Model file for the job. Use its own axes, mm. Face numbers are marked on the shaded views. A direction names the side the tool comes from. Coordinates: 2 decimals unless noted, no trailing zeros. Write each loop counter-clockwise with the first axis right and the second up, starting at its lowest first coordinate (ties: lowest second). Pieces come first, ordered by that corner, then holes. Notation, with made-up numbers: M 69.25,85 L 116.25,85 A25 ccw 116.25,100 Z; hole C -37.5,-13 d9. An arc over 180 degrees is marked long. Answer in a Markdown table with one row per item. Add a question column.
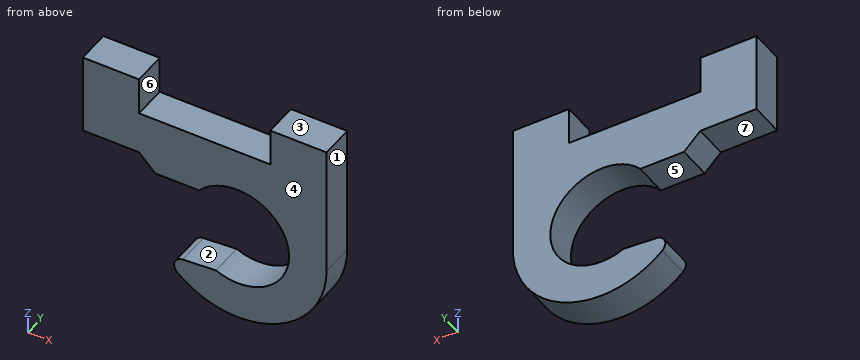
```python
from build123d import *

# Parameters (mm, degrees)
SKETCH1_R           = 2.75
BOSS_EXTRUDE1_DEPTH = 1.8
CUT_EXTRUDE1_DEPTH  = 1.8
FILLET1_R           = 0.5


with BuildPart() as part:
    # Sketch1 → Boss-Extrude1 (new body)
    with BuildSketch(Plane(origin=(0, 0, 0), x_dir=(1, 0, 0), z_dir=(0, 1, 0))):
        with BuildLine():
            Line((4.75, 0), (4.75, -5))
            Line((4.75, -5), (4.75, -7))
            Line((4.75, -7), (1.75, -7))
            Line((1.75, -7), (1.75, -5))
            Line((1.75, -5), (-5.25, -5))
            Line((-5.25, -5), (-5.25, -7))
            Line((-5.25, -7), (-8.25, -7))
            Line((-8.25, -7), (-8.25, -5))
            Line((-8.25, -5), (-8.25, -2.7))
            Line((-8.25, -2.7), (-5.25, -2.7))
            Line((-5.25, -2.7), (-4.382350157, -1.832350157))
            ThreePointArc((-4.382350157, -1.832350157), (-0.93443479, 4.657180652), (4.75, 0))
        make_face()
        Circle(SKETCH1_R, mode=Mode.SUBTRACT)
    extrude(amount=BOSS_EXTRUDE1_DEPTH)

    # Sketch2 → Cut-Extrude1 (cut)
    with BuildSketch(Plane(origin=(0, 1.8, 0), x_dir=(1, 0, 0), z_dir=(0, 1, 0))):
        Polygon((-5, 2.767649843), (0, 2.418015783), (0, -1.832350157), (-5, -1.832350157), align=None)
    extrude(amount=-CUT_EXTRUDE1_DEPTH, mode=Mode.SUBTRACT)

    # Fillet1
    fillet1_edges = [part.edges().sort_by_distance(p)[0] for p in [
        (-3.913732442, 0.9, -2.691690615),
    ]]
    fillet(fillet1_edges, radius=FILLET1_R)


solid = part.part
```
1) Drill centre lines: probe 1 along Z at (x, y) = (0, 1.2); probe 2 along X at (y, z) = (1.05, 0); probe 3 along Z at (x, y) = (-4, 0.25). Where is each one in solid material? Low to high.
2) Two-plate mould, pull along Z, no slides. Class the marked faces 1, 2 and 3: released by +Z, released by -Z, zero draft, split by the parting line, or undercut.
3) Slice it at C-C (y = 0.85). Give the cut face in (x, z), then the cut area to 3 significant figures.
4) Which spindle directions (+Z, -Z, +X, -X, +Y, -Y) get a long thin tool onto all of the face, cutting with end or side? Do the marked faces 4, 5, 6 and 7. Say none if no direction does.
5) Flat gauge pins, fed straight in: pin 1 Ø0.5 at (x, y) = (-3, 1) entering from -Z; pin 2 Ø3.5 at (x, z) = (0, 0) entering from +Y; pin 3 Ø0.5 at (x, y) = (-1.5, 1) entering from +Z; pin 4 Ø0.9 at (x, y) = (-7, 1) entering from -Z. Where does each tip first touch, or does it go through?
6) Slice it at A-A (z = 6). Give the cut face in (x, y).
7) Slice it at D-D (x = 3.25). Give the cut face in (y, z).
8) Slice it at B-B (x = 0). Give the cut face in (y, z), then the cut area to 3 significant figures.
Ans:
| question | item | result |
|---|---|---|
| 1 | probe 1 | z = -4.75 to -2.75, 2.75 to 5 |
| 1 | probe 2 | x = 2.75 to 4.75 |
| 1 | probe 3 | z = 1.83 to 5 |
| 2 | face 1 | zero draft |
| 2 | face 2 | undercut |
| 2 | face 3 | released by +Z |
| 3 | outline | M -8.25,2.7 L -5.25,2.7 L -4.38,1.83 L -2.05,1.83 A2.75 cw long -1.15,-2.5 L -2.92,-2.62 A0.5 ccw -3.22,-3.49 A4.75 ccw 4.75,0 L 4.75,7 L 1.75,7 L 1.75,5 L -5.25,5 L -5.25,7 L -8.25,7 Z |
| 3 | area | 69.2 mm2 |
| 4 | face 4 | +Z, -Z, +X, -X, -Y |
| 4 | face 5 | -X, +Y, -Y |
| 4 | face 6 | +Z, +Y, -Y |
| 4 | face 7 | -Z, -X, +Y, -Y |
| 5 | pin 1 | stops at z = -3.87 |
| 5 | pin 2 | passes through |
| 5 | pin 3 | stops at z = 5 |
| 5 | pin 4 | stops at z = 2.7 |
| 6 | outline | M -8.25,0 L -5.25,0 L -5.25,1.8 L -8.25,1.8 Z; M 1.75,0 L 4.75,0 L 4.75,1.8 L 1.75,1.8 Z |
| 7 | outline | M 0,-3.46 L 1.8,-3.46 L 1.8,7 L 0,7 Z |
| 8 | outline | M 0,-4.75 L 1.8,-4.75 L 1.8,-2.75 L 0,-2.75 Z; M 0,2.75 L 1.8,2.75 L 1.8,5 L 0,5 Z |
| 8 | area | 7.65 mm2 |
